Answer from the drawing. Dimensions are ordinates in mm from the lowest x, y and z of the part. Give positions to 0.01 mm unless a question says otherwise; leave off trailing zeros. Write each loop counter-clockwise with the first axis right and the second up, starting at its lowest first coordinate (ties: lowest second). Pieces come first, ordered by that corner, then holes. Notation, with made-up numbers: (40.5, -5) -> (93.5, -5) arc R12 ccw to (93.5, 9) -> close; hole circle Ø5 at (79.5, -24). An arc over 180 degrees is marked (long way). Put each result on its own line as item: value. Start each with the question number.
1) A cutting plane is placed at A-A (z = 1.25). Give the number of separate pieces and of enclosed holes in the cut face, then the cut area to 3 significant figures.
2) A cutting plane is placed at B-B (y = 6). Write down the section's boundary in (x, z), then the cut area to 3 significant figures.
3) Flat-ended cylindrical pins translate along their axes: pin 1 Ø1.5 at (x, y) = (155.5, 21) entering from -Z; pin 2 Ø2.5 at (x, y) = (171.45, 28.575) entering from +Z. Find the tip coordinate at first contact, or state that the pin passes through.
4) A cutting plane is placed at D-D (y = 34.5). Write down the section's boundary in (x, z), then the cut area to 3 significant figures.
5) A cutting plane is placed at C-C (x = 95.25). Write down the section's boundary in (y, z) (3 decimals).
6) Find the intervals of material crossed by line 1 along Y through (x, z) = (19, 5.5); line 2 along X through (y, z) = (29, 6.25) (3 decimals); line 3 along X through (y, z) = (9, 1.75), in increasing order. Write a range as from..to.
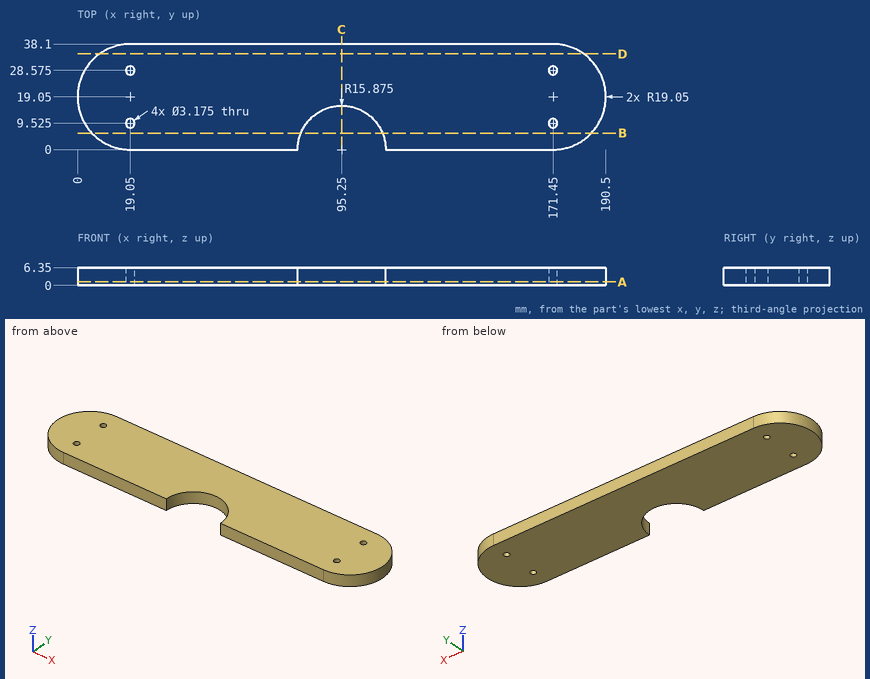
Reply:
1. separate pieces: 1
1. enclosed holes: 4
1. area: 6,520 mm2
2. outline: (5.17, 0) -> (80.55, 0) -> (80.55, 6.35) -> (5.17, 6.35) -> close; (109.95, 0) -> (185.33, 0) -> (185.33, 6.35) -> (109.95, 6.35) -> close
2. area: 957 mm2
3. pin 1: stops at z = 0
3. pin 2: passes through
4. outline: (7.91, 0) -> (182.59, 0) -> (182.59, 6.35) -> (7.91, 6.35) -> close
4. area: 1,110 mm2
5. outline: (15.875, 0) -> (38.1, 0) -> (38.1, 6.35) -> (15.875, 6.35) -> close
6. line 1: y = 0..7.94, 11.11..26.99, 30.16..38.1
6. line 2: x = 2.805..17.52, 20.58..169.92, 172.98..187.695
6. line 3: x = 2.87..17.55, 20.55..82.17, 108.33..169.95, 172.95..187.63
